CAD build for the part. Positions are in the model's coordinates, mm. Face numbers are marked on the shaded views. A direction names the side the tool comes from. Give positions to 0.01 mm unless a question says otherwise; leave off trailing zeros. Write each loop counter-clockwise with the first axis right and the second up, starting at its lowest first coordinate (ties: lowest second). Pieces come first, ordered by that corner, then holes. Notation, with made-up numbers: (8.25, 74.25) -> (55.25, 74.25) arc R24 cw to (55.25, 89.25) -> close; hole circle Ø5 at (86, 26.25). An arc over 180 degrees is marked (long way). Answer as a JSON object with one key per item and string values.
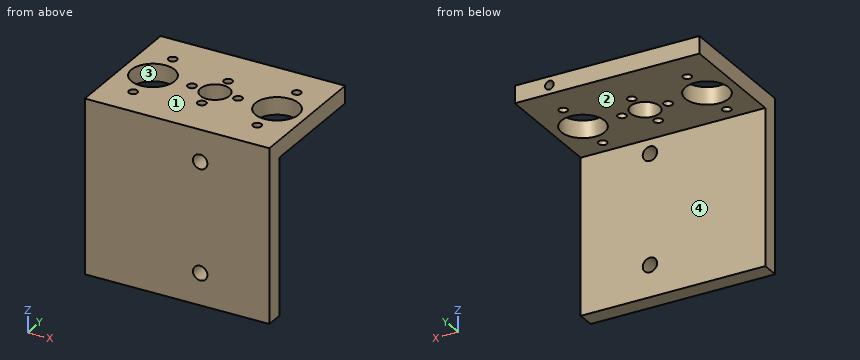
```python
from build123d import *

# Parameters (mm, degrees)
EXTRUDE_1_DEPTH     = 104
SKETCH_2_R          = 2.5
CUT_EXTRUDE_1_DEPTH = 151.638640461
SKETCH_3_R          = 5
SKETCH_3_R_2        = 1.5
SKETCH_3_R_3        = 7.5
CUT_EXTRUDE_2_DEPTH = 142.887279204
SKETCH_4_R          = 1.5
CUT_EXTRUDE_3_DEPTH = 5


with BuildPart() as part:
    # 草图1 → 凸台-拉伸1 (new body)
    with BuildSketch(Plane(origin=(0, 0, 0), x_dir=(0, 0, -1), z_dir=(1, 0, 0))):
        Polygon((0, 0), (80, 0), (80, 6), (6, 6), (6, 80), (0, 80), (0, 6), align=None)
    extrude(amount=EXTRUDE_1_DEPTH)

    # 草图2 → 切除-拉伸1 (cut, through all)
    with BuildSketch(Plane(origin=(0, 6, 0), x_dir=(1, 0, 0), z_dir=(0, 1, 0))):
        with Locations(Location((60, 11, 0), (0, 0, 270))):
            Circle(SKETCH_2_R)
        with Locations(Location((60, 49, 0), (0, 0, 270))):
            Circle(SKETCH_2_R)
        Polygon((84, 60), (20, 60), (20, 6), (0, 6), (0, 80), (84, 80), (104, 80), (104, 6), (84, 6), align=None)
    extrude(amount=-CUT_EXTRUDE_1_DEPTH, mode=Mode.SUBTRACT)

    # 草图3 → 切除-拉伸2 (cut, through all)
    with BuildSketch(Plane(origin=(0, 0, -6), x_dir=(-1, 0, 0), z_dir=(0, 0, -1))):
        with Locations((-52, 23)):
            Circle(SKETCH_3_R)
        with Locations((-52, 15)):
            Circle(SKETCH_3_R_2)
        with Locations((-60, 23)):
            Circle(SKETCH_3_R_2)
        with Locations((-52, 31)):
            Circle(SKETCH_3_R_2)
        with Locations((-44, 23)):
            Circle(SKETCH_3_R_2)
        with Locations((-30.5, 23)):
            Circle(SKETCH_3_R_3)
        with Locations((-30.5, 35)):
            Circle(SKETCH_3_R_2)
        with Locations(Location((-30.5, 11, 0), (0, 0, 180))):
            Circle(SKETCH_3_R_2)
        with Locations((-73.5, 11)):
            Circle(SKETCH_3_R_2)
        with Locations(Location((-73.5, 23, 0), (0, 0, 180))):
            Circle(SKETCH_3_R_3)
        with Locations(Location((-73.5, 35, 0), (0, 0, 180))):
            Circle(SKETCH_3_R_2)
        Polygon((-84, 0), (-84, 46), (-20, 46), (-20, 0), (0, 0), (0, 80), (-104, 80), (-104, 0), align=None)
    extrude(amount=-CUT_EXTRUDE_2_DEPTH, mode=Mode.SUBTRACT)

    # 草图4 → 切除-拉伸3 (cut)
    with BuildSketch(Plane(origin=(0, 46, 0), x_dir=(1, 0, 0), z_dir=(0, 1, 0))):
        with Locations(Location((72, 3, 0), (0, 0, 270))):
            Circle(SKETCH_4_R)
    extrude(amount=-CUT_EXTRUDE_3_DEPTH, mode=Mode.SUBTRACT)


solid = part.part
```
1) Wall check: probe 1 along Y at (x, z) = (30.5, -1.45); probe 2 along Y at (x, z) = (52, -1.6); probe 3 along X at (y, z) = (4.55, -49). Give the ranges that are in metal, low to high.
Model answer:
{"probe 1": "y = 0 to 9.5, 12.5 to 15.5, 30.5 to 33.5, 36.5 to 46", "probe 2": "y = 0 to 13.5, 16.5 to 18, 28 to 29.5, 32.5 to 46", "probe 3": "x = 20 to 57.5, 62.5 to 84"}
2) Mould opens along X. For the marked faces 3 and 4 say: released by +X, released by -X, zero draft, split by the parting line, or undercut.
Model answer:
{"face 3": "undercut", "face 4": "zero draft"}
3) Slice it at D-D (z = -3). State how many separate pieces and enclosed holes the cut face has, then the cut area to 3 significant figures.
Model answer:
{"separate pieces": "1", "enclosed holes": "11", "area": "2,440 mm2"}
4) Slice it at A-A (y = 11). List the corners of the cut face in (x, z).
Model answer:
{"outline": "(20, -6) -> (29, -6) -> (29, 0) -> (20, 0) -> close; (32, -6) -> (72, -6) -> (72, 0) -> (32, 0) -> close; (75, -6) -> (84, -6) -> (84, 0) -> (75, 0) -> close"}
5) Slice it at B-B (z = -49). List the corners of the cut face in (x, y).
Model answer:
{"outline": "(20, 0) -> (57.5, 0) -> (57.5, 6) -> (20, 6) -> close; (62.5, 0) -> (84, 0) -> (84, 6) -> (62.5, 6) -> close"}
6) Slice it at C-C (x = 60). List the corners of the cut face in (y, z), then the cut area to 3 significant figures.
Model answer:
{"outline": "(0, -60) -> (6, -60) -> (6, -51.5) -> (0, -51.5) -> close; (0, -46.5) -> (6, -46.5) -> (6, -13.5) -> (0, -13.5) -> close; (0, -8.5) -> (6, -8.5) -> (6, -6) -> (21.5, -6) -> (21.5, 0) -> (0, 0) -> close; (24.5, -6) -> (46, -6) -> (46, 0) -> (24.5, 0) -> close", "area": "522 mm2"}
7) 3-axis set-ups, long thin cutter, end or side, ignore diameter. For the marked faces 1 and 2: which of +Z, -Z, +X, -X, +Y, -Y reach the whole face in a straight line?
Model answer:
{"face 1": "+Z, +X, -X, +Y, -Y", "face 2": "-Z, +X, -X, +Y"}
8) Pin check, flat tips, straight feed: pin 1 (6 mm diameter, centred on x = 50, y = 15.5, fed in from +Z); pin 2 (3.5 mm diameter, centred on x = 73.5, y = 35, fed in from -Z); pin 3 (16 mm diameter, centred on x = 64, z = -21.5, fed in from +Y); pin 4 (0.9 mm diameter, centred on x = 72.5, z = -3, fed in from +Y). Stop position of each tip, or through.
Model answer:
{"pin 1": "stops at z = 0", "pin 2": "stops at z = -6", "pin 3": "stops at y = 6", "pin 4": "stops at y = 41"}
